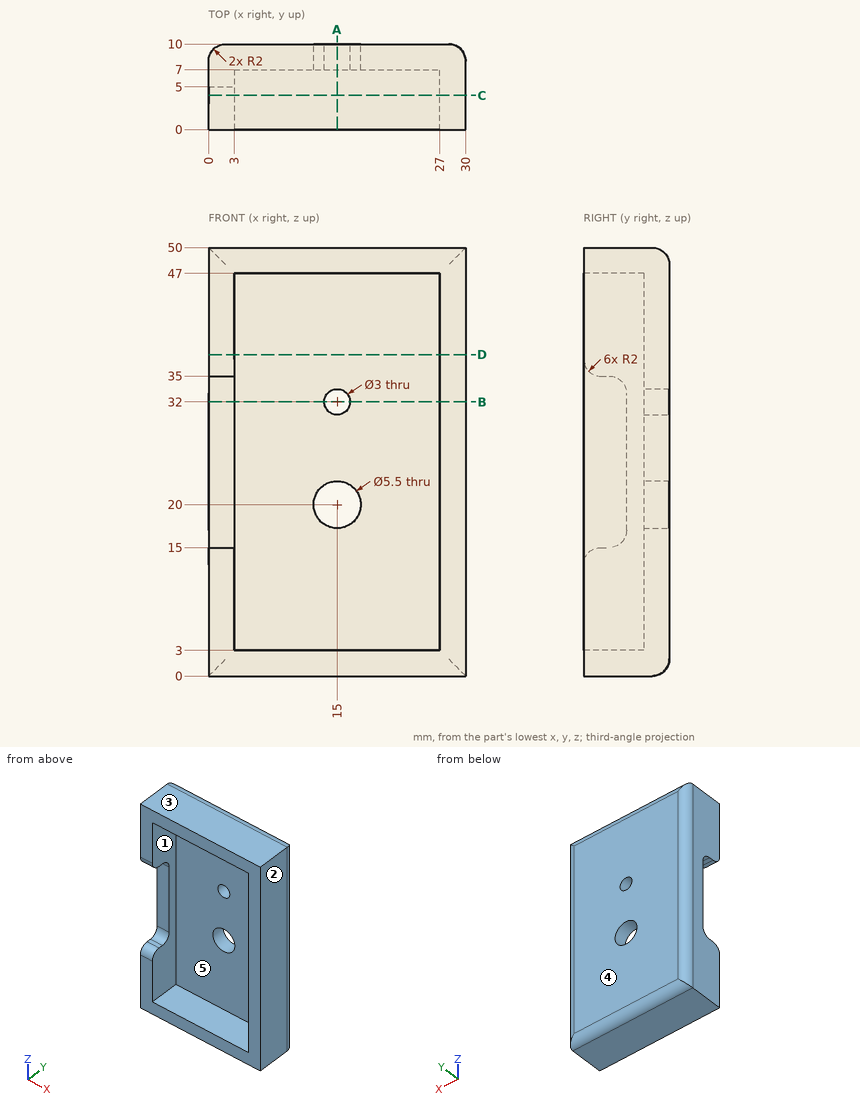
Geometry check sheet. Reference: drawing and pictorial views, mm from the part's lowest x, y, z. A direction names the side the tool comes from. Coordinates: 2 decimals unless noted, no trailing zeros. Order: outer loops, then holes, each group sorted by start corner. A loop starts at its lowest first (then second) coordinate and runs counter-clockwise, first axis right, second up. Notation, with made-up numbers: (60.5, 46.5) -> (93.5, 46.5) arc R25 ccw to (93.5, 62.5) -> close; hole circle Ø10 at (88.25, -9.5). An arc over 180 degrees is marked (long way). Use CSV: the item, a comma, the result in double quotes. Start each with the question number.
Q1. Tool access check on the marked faces 1 and 2. Record the directions out of +Z, -Z, +X, -X, +Y, -Y that give a thin tool (end or side, any length) a straight path to the whole face; none if there is none.
Q2. Depth check by flat-ended pin: P1, Ø7, axis at x = 15, z = 20, coming from the -Y side; P2, Ø3.5, axis at x = 1, z = 21.5, coming from the -Y side; P3, Ø3, axis at y = 1.5, z = 16.5, coming from the -X side. Enter the tip coordinate at first touch or a pass-through.
Q3. Section check A-A, the plane x = 15. Record the cut outline in (y, z), and give its area (3 significant figures).
Q4. Section check D-D, the plane z = 37.5. Record the cut outline in (x, y), and give its area (3 significant figures).
Q5. Section check B-B, the plane z = 32. Record the cut outline in (x, y), and give its area (3 significant figures).
Q6. Section check C-C, the plane y = 4. Record the cut outline in (x, z), and give its area (3 significant figures).
Q7. Draft check along Z on the marked faces 3, 4 and 5. Enter one of: +Z half, -Z half, draft (parallel to the pull), parting line (faces both ways), or undercut.
Q8. Thickness scan on line 1 along Z through (x, y) = (16.75, 1.25); line 2 along X through (y, z) = (6, 27); line 3 along Y through (x, z) = (23.75, 20). Record the ranges inside material, lowest first.
Returned:
1,face 1,"-Y"
1,face 2,"+Z, -Z, +X, +Y, -Y"
2,P1,"stops at y = 7"
2,P2,"stops at y = 5"
2,P3,"stops at x = 27"
3,outline,"(0, 0) -> (8, 0) arc R2 ccw to (10, 2) -> (10, 17.25) -> (7, 17.25) -> (7, 3) -> (0, 3) -> close; (0, 47) -> (7, 47) -> (7, 33.5) -> (10, 33.5) -> (10, 48) arc R2 ccw to (8, 50) -> (0, 50) -> close; (7, 22.75) -> (10, 22.75) -> (10, 30.5) -> (7, 30.5) -> close"
3,area,"165 mm^2"
4,outline,"(0, 0) -> (3, 0) -> (3, 7) -> (27, 7) -> (27, 0) -> (30, 0) -> (30, 8) arc R2 ccw to (28, 10) -> (2, 10) arc R2 ccw to (0, 8) -> close"
4,area,"130 mm^2"
5,outline,"(0, 5) -> (3, 5) -> (3, 7) -> (13.5, 7) -> (13.5, 10) -> (2, 10) arc R2 ccw to (0, 8) -> close; (16.5, 7) -> (27, 7) -> (27, 0) -> (30, 0) -> (30, 8) arc R2 ccw to (28, 10) -> (16.5, 10) -> close"
5,area,"106 mm^2"
6,outline,"(0, 0) -> (30, 0) -> (30, 50) -> (0, 50) -> (0, 34.73) -> (3, 34.73) -> (3, 47) -> (27, 47) -> (27, 3) -> (3, 3) -> (3, 15.27) -> (0, 15.27) -> close"
6,area,"386 mm^2"
7,face 3,"+Z half"
7,face 4,"draft"
7,face 5,"undercut"
8,line 1,"z = 0 to 3, 47 to 50"
8,line 2,"x = 0 to 3, 27 to 30"
8,line 3,"y = 7 to 10"
